```python
from build123d import *

# Parameters (mm, degrees)
SKETCH2_R           = 8.2
BOSS_EXTRUDE1_DEPTH = 166
SKETCH3_R           = 2.1
CUT_EXTRUDE1_DEPTH  = 10
CUT_EXTRUDE2_START  = -10
SKETCH4_R           = 2.1
CUT_EXTRUDE2_DEPTH  = 10


with BuildPart() as part:
    # Sketch2 → Boss-Extrude1 (new body)
    with BuildSketch(Plane(origin=(0, 0, 0), x_dir=(1, 0, 0), z_dir=(0, 1, 0))):
        with Locations(Location((0, 0, 0), (0, 0, 270))):
            Circle(SKETCH2_R)
    extrude(amount=BOSS_EXTRUDE1_DEPTH)

    # Sketch3 → Cut-Extrude1 (cut)
    with BuildSketch(Plane(origin=(0, 166, 0), x_dir=(1, 0, 0), z_dir=(0, 1, 0))):
        with Locations(Location((0, 0, 0), (0, 0, 270))):
            Circle(SKETCH3_R)
    extrude(amount=-CUT_EXTRUDE1_DEPTH, mode=Mode.SUBTRACT)

    # Sketch4 → Cut-Extrude2 (cut)
    with BuildSketch(Plane.XZ.offset(CUT_EXTRUDE2_START)):
        with Locations(Location((0, 0, 0), (0, 0, 90))):
            Circle(SKETCH4_R)
    extrude(amount=CUT_EXTRUDE2_DEPTH, mode=Mode.SUBTRACT)


solid = part.part
```
Check sheet for the modelled part. Datum: model origin and axes. Units: mm. A direction names the side the tool comes from. Round coordinates to 2 decimals unless told otherwise and drop trailing zeros. Loops run counter-clockwise (first coordinate to the right, second up) from the corner with the lowest first, then second, coordinate; pieces in that order, holes last. Notation, with made-up numbers: M 44,56 L 91,56 A19 cw 91,78 Z; hole C 38,-3.5 d5. An arc over 180 degrees is marked long. Answer as a JSON object with one key per item and string values.
1. Mould release check, pull along X, two halves, no side actions. Record for faces 4 (the flat face through (0, 156, 0)), 5 (the cylindrical face through (8.13, 81.84, -1.07)), 6 (the cylindrical face through (-0.631, 5.07, 2.003)), 7 (the flat face through (-2, 166, 2)): pulls with the +X half, pulls with the -X half, needs draft (parallel to the pull), parting line crosses it, or undercut.
Reply:
{"face 4": "undercut", "face 5": "parting line crosses it", "face 6": "undercut", "face 7": "needs draft"}
2. Access from +Z, -Z, +X, -X, +Y, -Y to the whole of each face (thin tool, end or side, straight path). Record for faces 1 (the flat face through (-2, 0, 2)), 2 (the cylindrical face through (0.631, 161.07, 2.003)), 3 (the flat face through (0, 10, 0)).
Reply:
{"face 1": "+Z, -Z, +X, -X, -Y", "face 2": "+Y", "face 3": "-Y"}
3. Section check C-C (y = 130). Record the boundary of the cut face in (x, z).
Reply:
{"outline": "C 0,0 d16.4"}
4. Scan lines: line 1 (X direction, y = 5.25, z = 0); line 2 (Y direction, x = -2, z = 0.25); line 3 (X direction, y = 94.5, z = 0.25). Record each from-to range of solid material in increasing order.
Reply:
{"line 1": "x = -8.2 to -2.1, 2.1 to 8.2", "line 2": "y = 10 to 156", "line 3": "x = -8.2 to 8.2"}
5. Section check A-A (x = 0). Record the boundary of the cut face in (y, z), plus the area to 3 significant figures.
Reply:
{"outline": "M 0,-8.2 L 166,-8.2 L 166,-2.1 L 156,-2.1 L 156,2.1 L 166,2.1 L 166,8.2 L 0,8.2 L 0,2.1 L 10,2.1 L 10,-2.1 L 0,-2.1 Z", "area": "2,640 mm²"}
6. Section check B-B (z = 0). Record the boundary of the cut face in (x, y).
Reply:
{"outline": "M -8.2,0 L -2.1,0 L -2.1,10 L 2.1,10 L 2.1,0 L 8.2,0 L 8.2,166 L 2.1,166 L 2.1,156 L -2.1,156 L -2.1,166 L -8.2,166 Z"}
7. Gauge pin test, flat ends, axial feed: P1, Ø4, axis at x = -5, y = 41, coming from the +Z side; P2, Ø1.3, axis at x = 0.5, z = 0, coming from the -Y side; P3, Ø1.5, axis at y = 144, z = -6, coming from the +X side. Record the tip position at first contact, or that the pin passes through.
Reply:
{"P1": "stops at z = 7.63", "P2": "stops at y = 10", "P3": "stops at x = 6.3"}
